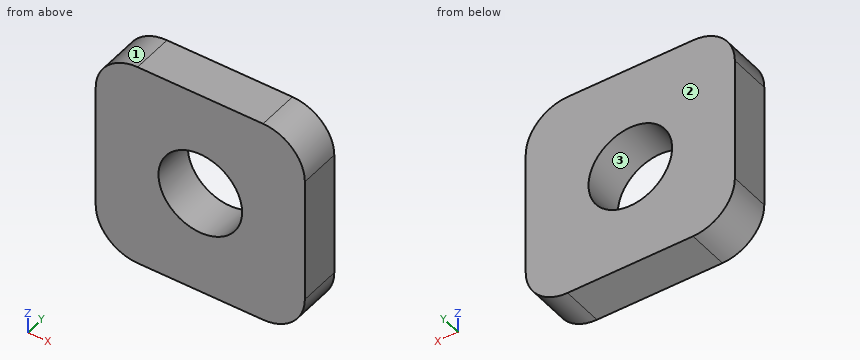
from build123d import *

# Parameters (mm, degrees)
F0_R     = 12.7
F1_DEPTH = 12.7


with BuildPart() as f1:
    # F0 (on Front) → F1 (new body)
    with BuildSketch(Plane.XZ):
        with BuildLine():
            ThreePointArc((31.75, 19.05), (28.030256, 28.030256), (19.05, 31.75))
            Line((19.05, 31.75), (-19.05, 31.75))
            ThreePointArc((-19.05, 31.75), (-28.030256, 28.030256), (-31.75, 19.05))
            Line((-31.75, 19.05), (-31.75, -19.05))
            ThreePointArc((-31.75, -19.05), (-28.030256, -28.030256), (-19.05, -31.75))
            Line((-19.05, -31.75), (19.05, -31.75))
            ThreePointArc((19.05, -31.75), (28.030256, -28.030256), (31.75, -19.05))
            Line((31.75, -19.05), (31.75, 19.05))
        make_face()
        Circle(F0_R, mode=Mode.SUBTRACT)
    extrude(amount=F1_DEPTH)


solid = f1.part
Design review of the part built by this model. Coordinates are the model's own, in mm. Face numbers are marked on the shaded views. Coordinates: 2 decimals unless noted, no trailing zeros. Loops run counter-clockwise (first coordinate to the right, second up) from the corner with the lowest first, then second, coordinate; pieces in that order, holes last.
Item 1: Clearance check with a flat-ended pin moving along its axis: pin 1 (23 mm diameter, centred on x = 0, z = 0, fed in from -Y). State where the tip first meets the part, or that it passes through.
Completed:
pin 1: passes through
Item 2: Add section C-C (x = 0). Write out the cut boundary in (y, z), and give its area (3 significant figures).
Completed:
outline: (-12.7, -31.75) - (0, -31.75) - (0, -12.7) - (-12.7, -12.7) - close; (-12.7, 12.7) - (0, 12.7) - (0, 31.75) - (-12.7, 31.75) - close
area: 484 mm2
Item 3: Draft analysis for pull direction Z (two halves, no side actions). For the marked faces 1, 2 and 3, state which applies: pulls with the +Z half, pulls with the -Z half, needs draft (parallel to the pull), parting line crosses it, or undercut.
Completed:
face 1: pulls with the +Z half
face 2: needs draft
face 3: undercut
Item 4: Wall thickness on L1, parallel to Z at x = 0, y = -5; L2, parallel to X at y = -9.25, z = 8.5; L3, parallel to X at y = -7.75, z = 5: over which ranges is each line inside the solid? List them lowest first.
Completed:
L1: z = -31.75 to -12.7, 12.7 to 31.75
L2: x = -31.75 to -9.44, 9.44 to 31.75
L3: x = -31.75 to -11.67, 11.67 to 31.75
Item 5: Add section A-A (y = -3.5). Write out the cut boundary in (x, z), and give its area (3 significant figures).
Completed:
outline: (-31.75, -19.05) arc R12.7 ccw to (-19.05, -31.75) - (19.05, -31.75) arc R12.7 ccw to (31.75, -19.05) - (31.75, 19.05) arc R12.7 ccw to (19.05, 31.75) - (-19.05, 31.75) arc R12.7 ccw to (-31.75, 19.05) - close; hole circle Ø25.4 at (0, 0)
area: 3,390 mm2
Item 6: Add section B-B (z = 0). Write out the cut boundary in (x, y), and give its area (3 significant figures).
Completed:
outline: (-31.75, -12.7) - (-12.7, -12.7) - (-12.7, 0) - (-31.75, 0) - close; (12.7, -12.7) - (31.75, -12.7) - (31.75, 0) - (12.7, 0) - close
area: 484 mm2
